Read the model definition and answer for the solid it produces. Units are mm, in the model's axes. Face numbers are marked on the shaded views. A direction names the side the tool comes from. Coordinates: 2 decimals unless noted, no trailing zeros. Order: outer loops, then holes, each group sorted by start corner. A loop starts at its lowest first (then second) coordinate and runs counter-clockwise, first axis right, second up.
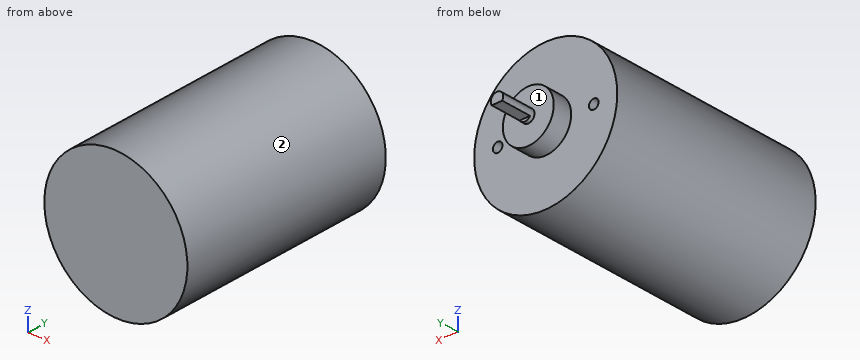
Autodesk Inventor part; units mm, degrees
ref_plane "YZ Plane" through (0, 0, 0) normal (1, 0, 0) x (0, 1, 0)
ref_plane "XZ Plane" through (0, 0, 0) normal (0, 1, 0) x (-1, 0, 0)
ref_plane "XY Plane" through (0, 0, 0) normal (0, 0, 1) x (1, 0, 0)
sketch "Sketch1" plane through (0, 0, 0) normal (0, 1, 0) x (-1, 0, 0)
  circle A0 centre (0, 0) radius 18.625
  dimension "d0" = 37.25
extrude "Extrusion1" add sketch "Sketch1" along normal blind 57
sketch "Sketch2" plane through (0, 57, 0) normal (0, 1, 0) x (1, 0, 0)
  circle A0 centre (0, 0) radius 6.625
  dimension "d3" = 13.25
extrude "Extrusion2" add sketch "Sketch2" along normal blind 5
sketch "Sketch3" plane through (0, 62, 0) normal (0, 1, 0) x (1, 0, 0)
  circle A0 centre (0, 0) radius 1.625
  dimension "d6" = 3.25
extrude "Extrusion3" add sketch "Sketch3" along normal blind 9
sketch "Sketch4" plane through (0, 71, 0) normal (0, 1, 0) x (1, 0, 0)
  circle A0 centre (0, 0) radius 1.625
  line L0 (0, 0.875) -> (-1.3693, 0.875)
  line L1 (0, 0.875) -> (1.3693, 0.875)
  arc A1 (1.3693, 0.875) -> (-1.3693, 0.875) centre (0, 0) ccw
extrude "Extrusion4" cut sketch "Sketch4" against normal blind 8 contours L1 L0 A0 picked at (0.8372, 0.9686)
sketch "Sketch5" plane through (0, 57, 0) normal (0, 1, 0) x (1, 0, 0)
  circle A0 centre (12.5, 0) radius 1.25
  circle A1 centre (-12.5, 0) radius 1.25
  line L0 (-12.5, 0) -> (0, 0)
  line L1 (0, 0) -> (12.5, 0)
  dimension "d13" = 2.5
  dimension "d14" = 2.5
  dimension "d17" = 12.5
  dimension "d18" = 12.5
extrude "Extrusion5" cut sketch "Sketch5" against normal blind 8
properties part number "Helion_Motor"
1) Straight lines are drawn through the part: line 1 (Y direction, x = -14.5, z = -7.5); line 2 (Z direction, x = -12.5, y = 54.5); line 3 (Z direction, x = 12, y = 53). For each, find the intervals that lie inside material, in ascending order.
A:
line 1: y = 0 to 57
line 2: z = -13.81 to -1.25, 1.25 to 13.81
line 3: z = -14.24 to -1.15, 1.15 to 14.24
2) A cutting plane is placed at D-D, the plane y = 9. Determine the outline of the cut face in (x, z) (3 decimals).
A:
outline: circle Ø37.25 at (0, 0)
3) A cutting plane is placed at C-C, the plane z = 0. Determine the outline of the cut face in (x, y) (3 decimals), and give its area (3 significant figures).
A:
outline: (-18.625, 0) - (18.625, 0) - (18.625, 57) - (13.75, 57) - (13.75, 49) - (11.25, 49) - (11.25, 57) - (6.625, 57) - (6.625, 62) - (1.625, 62) - (1.625, 71) - (-1.625, 71) - (-1.625, 62) - (-6.625, 62) - (-6.625, 57) - (-11.25, 57) - (-11.25, 49) - (-13.75, 49) - (-13.75, 57) - (-18.625, 57) - close
area: 2,180 mm2
4) Flat-ended cylindrical pins translate along their axes: pin 1 Ø3 at (x, z) = (-8.5, 13.5) entering from +Y; pin 2 Ø2 at (x, z) = (-12.5, 0) entering from +Y; pin 3 Ø4 at (y, z) = (63.5, -1.5) entering from -X. Find the tip coordinate at first contact, or state that the pin passes through.
A:
pin 1: stops at y = 57
pin 2: stops at y = 49
pin 3: stops at x = -6.62
5) A cutting plane is placed at B-B, the plane y = 54.5. Determine the outline of the cut face in (x, z) (3 decimals).
A:
outline: circle Ø37.25 at (0, 0); hole circle Ø2.5 at (-12.5, 0); hole circle Ø2.5 at (12.5, 0)
6) A cutting plane is placed at A-A, the plane x = 0. Determine the outline of the cut face in (y, z) (3 decimals), and give its area (3 significant figures).
A:
outline: (0, -18.625) - (57, -18.625) - (57, -6.625) - (62, -6.625) - (62, -1.625) - (63, -1.625) - (63, -0.875) - (71, -0.875) - (71, 1.625) - (62, 1.625) - (62, 6.625) - (57, 6.625) - (57, 18.625) - (0, 18.625) - close
area: 2,210 mm2
7) Which of the six approach directions +Z, -Z, +X, -X, +Y, -Y give full straight-line access (tool end or side, diameter ignored) to the marked faces 1 and 2?
A:
face 1: +Y
face 2: +Y, -Y
